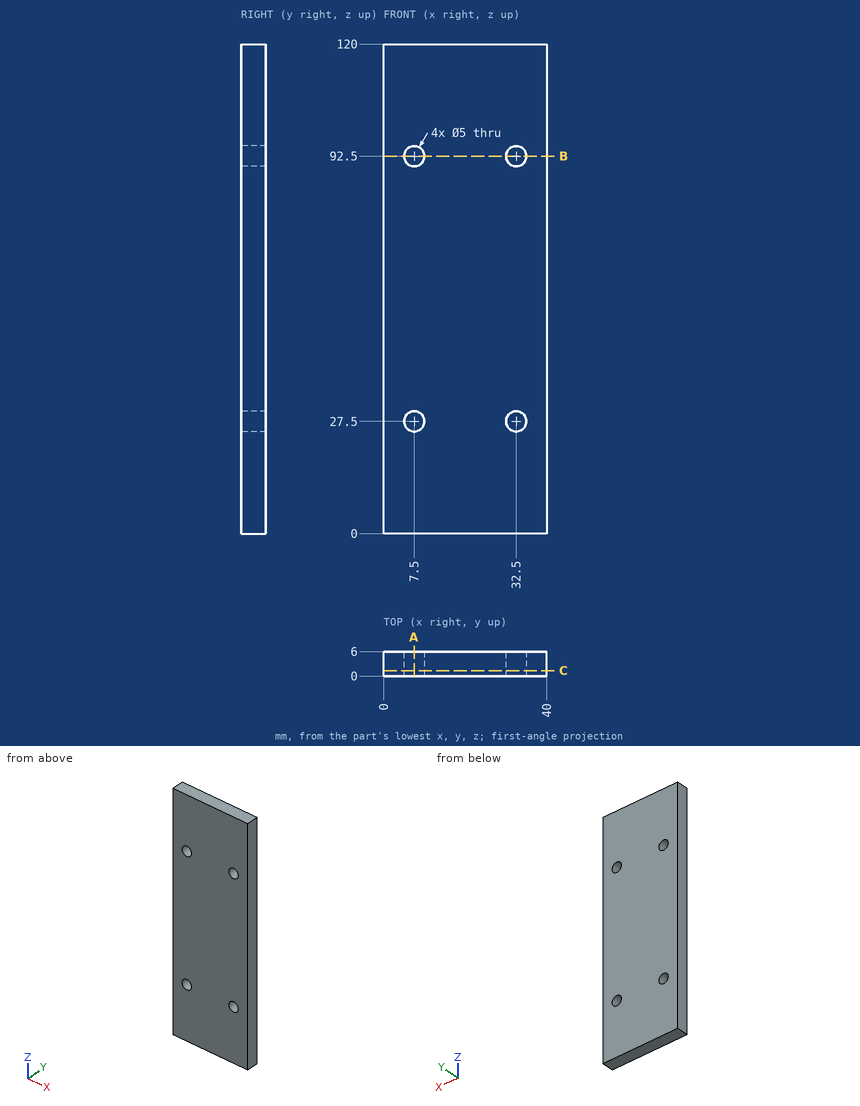
Design review of the part shown in the three views and the two pictorial views. Dimensions are in mm from the part's minimum x, y and z. Coordinates: 2 decimals unless noted, no trailing zeros. Order: outer loops, then holes, each group sorted by start corner. A loop starts at its lowest first (then second) coordinate and runs counter-clockwise, first axis right, second up.
Item 1: For pin 1 Ø6 at (x, z) = (7.5, 92.5) entering from +Y, flat-tipped, find the tip position at first contact; note if it passes through.
Item 2: Take a section at B-B, the plane z = 92.5. Write out the cut boundary in (x, y).
Item 3: Take a section at A-A, the plane x = 7.5. Write out the cut boundary in (y, z), then the cut area to 3 significant figures.
Item 4: Take a section at C-C, the plane y = 1.3. Write out the cut boundary in (x, z), then the cut area to 3 significant figures.
Item 5: For line 1 (Z direction, x = 7.5, y = 4.65); line 2 (X direction, y = 2.4, z = 92.5); line 3 (Z direction, x = 6, y = 3.15), list the stretches that pass through material, from the lowest coordinate up.
The answers:
1. pin 1: stops at y = 6
2. outline: (0, 0) - (5, 0) - (5, 6) - (0, 6) - close; (10, 0) - (30, 0) - (30, 6) - (10, 6) - close; (35, 0) - (40, 0) - (40, 6) - (35, 6) - close
3. outline: (0, 0) - (6, 0) - (6, 25) - (0, 25) - close; (0, 30) - (6, 30) - (6, 90) - (0, 90) - close; (0, 95) - (6, 95) - (6, 120) - (0, 120) - close
3. area: 660 mm2
4. outline: (0, 0) - (40, 0) - (40, 120) - (0, 120) - close; hole circle Ø5 at (7.5, 27.5); hole circle Ø5 at (7.5, 92.5); hole circle Ø5 at (32.5, 27.5); hole circle Ø5 at (32.5, 92.5)
4. area: 4,720 mm2
5. line 1: z = 0 to 25, 30 to 90, 95 to 120
5. line 2: x = 0 to 5, 10 to 30, 35 to 40
5. line 3: z = 0 to 25.5, 29.5 to 90.5, 94.5 to 120
